Source: CAD feature listing. Evaluate the final solid. Frame: model axes, mm. A direction names the side the tool comes from. Give positions to 0.01 mm unless a question says otherwise; leave off trailing zeros. Loops run counter-clockwise (first coordinate to the right, second up) from the corner with the lowest first, then second, coordinate; pieces in that order, holes last. Notation, with made-up numbers: (-30.5, 4) - (6.5, 4) arc R19 ccw to (6.5, 18) - close; hole circle Ø9 at (-32.75, -12.5). An arc over 180 degrees is marked (long way). Put each result on its own line as item: value.
```python
from build123d import *

# Parameters (mm, degrees)
F3_DEPTH = 5
F4_R     = 0.8


with BuildPart() as f1:
    # F0 (on Front) → F1 (revolve)
    with BuildSketch(Plane.XZ):
        Polygon((0, 12.72551), (0, 0), (33, 0), (33, 5), (8, 5), align=None)
    revolve(axis=Axis((16.5, 0, 0), (-1, 0, 0)))

    # F2 (on face) → F3 (cut)
    with BuildSketch(Plane(origin=(0, 0, 0), x_dir=(0, -1, 0), z_dir=(-1, 0, 0))):
        Polygon((3.996034, 4.167138), (-1.610831, 5.544236), (-5.606865, 1.377098), (-3.996034, -4.167138), (1.610831, -5.544236), (5.606865, -1.377098), align=None)
    extrude(amount=-F3_DEPTH, mode=Mode.SUBTRACT)

    # F4
    f4_edges = [f1.edges().sort_by_distance(p)[0] for p in [
        (33, 0, -5),
    ]]
    fillet(f4_edges, radius=F4_R)


solid = f1.part
```
1) Section query C-C, the plane z = 0. Output: boundary loops of the cut face in (x, y).
Check result:
outline: (0, -12.73) - (8, -5) - (32.2, -5) arc R0.8 ccw to (33, -4.2) - (33, 4.2) arc R0.8 ccw to (32.2, 5) - (8, 5) - (0, 12.73) - (0, 5.21) - (5, 5.21) - (5, -5.21) - (0, -5.21) - close
2) Mould query, pull axis Z, two halves, no side actions, for faces 4 (the conical face through (7.5, -5.35, -1.19)), 5 (the flat face through (33, 0, 0)), 6 (the flat face through (2.5, 4.8, -1.4)). Classes: pulls with the +Z half, pulls with the -Z half, needs draft (parallel to the pull), parting line crosses it, or undercut.
Check result:
face 4: parting line crosses it
face 5: needs draft
face 6: undercut
3) Section query D-D, the plane x = 11.5. Output: boundary loops of the cut face in (y, z), plus the area to 3 significant figures.
Check result:
outline: circle Ø10 at (0, 0)
area: 78.5 mm²
4) Section query A-A, the plane x = 2.5. Output: boundary loops of the cut face in (y, z), plus the area to 3 significant figures.
Check result:
outline: circle Ø20.62 at (0, 0); hole (-5.61, -1.38) - (-1.61, -5.54) - (4, -4.17) - (5.61, 1.38) - (1.61, 5.54) - (-4, 4.17) - close
area: 247 mm²
5) Pin query (flat end, axial travel): P1, Ø12, axis at x = 29.5, z = 10, coming from the -Y side; P2, Ø8, axis at x = 4.5, y = -4.5, coming from the -Z side; P3, Ø1, axis at x = 7, z = -0.5, coming from the -Y side. Return the tip coordinate at first contact, or that it passes through.
Check result:
P1: y = -3
P2: z = -11.61
P3: y = -6.43
6) Access query for faces 1 (the cylindrical face through (19.93, -4.88, -1.08)), 2 (the flat face through (0, 0.2, 5.5)), 3 (the flat face through (2.465, 1.232, -4.846)). Directions: +Z, -Z, +X, -X, +Y, -Y. A direction counts if a zero-diameter tool reaches every point of the face in a straight line with its end or side. Return the directions, or none.
Check result:
face 1: +X
face 2: +Z, -Z, -X, +Y, -Y
face 3: -X
7) Material intervals for line 1 along X through (y, z) = (2, -2); line 2 along Z through (x, y) = (15, -0.25); line 3 along X through (y, z) = (7.25, 0), sorted ascending. Write a range as [from, to].
Check result:
line 1: [5, 33]
line 2: [-4.99, 4.99]
line 3: [0, 5.67]
8) Section query B-B, the plane y = 0. Output: boundary loops of the cut face in (x, z), plus the area to 3 significant figures.
Check result:
outline: (0, -12.73) - (8, -5) - (32.2, -5) arc R0.8 ccw to (33, -4.2) - (33, 4.2) arc R0.8 ccw to (32.2, 5) - (8, 5) - (0, 12.73) - (0, 5.15) - (5, 5.15) - (5, -5.15) - (0, -5.15) - close
area: 340 mm²
